The drawing under review shows one solid part. Ordinate dimensions are in mm from its lowest x, y, z. A direction names the side the tool comes from. Coordinates: 2 decimals unless noted, no trailing zeros. Order: outer loops, then holes, each group sorted by start corner. A loop starts at its lowest first (then second) coordinate and runs counter-clockwise, first axis right, second up. Notation, with made-up numbers: M 26.5,49.25 L 41.5,49.25 A26 ccw 41.5,70.25 Z; hole C 29.25,80.5 d2. An arc over 180 degrees is marked long. Answer as a JSON object with one key per item and string values.
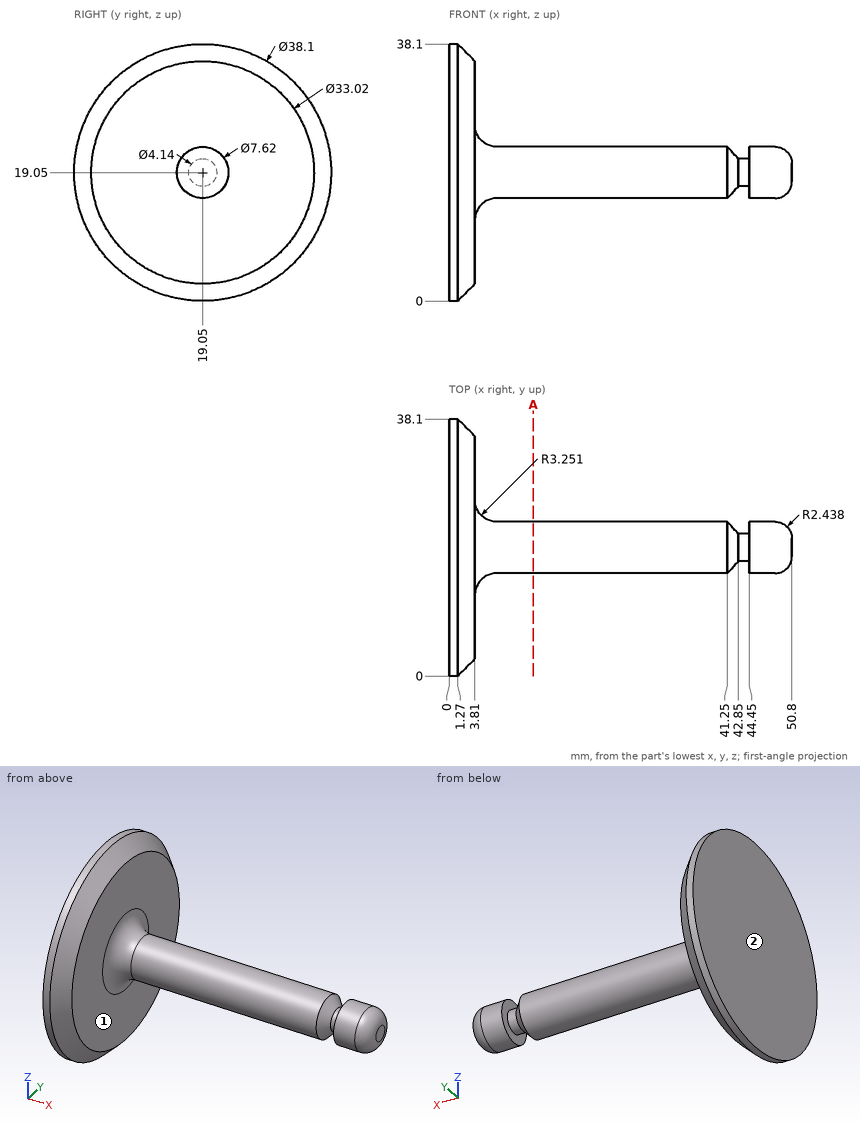
1) To check wall thickness, follow L1, parallel to X at y = 19.5, z = 34; L2, parallel to Z at x = 41, y = 19; L3, parallel to X at y = 24, z = 19. State the ranges of each line that lie inside material, in increasing order.
Taken from the geometry:
{"L1": "x = 0 to 3.81", "L2": "z = 15.24 to 22.86", "L3": "x = 0 to 4.59"}
2) Tool access review of the marked faces 1 and 2: name each direction out of +Z, -Z, +X, -X, +Y, -Y from which nothing blocks a thin tool from reaching the whole face with its end or side.
Taken from the geometry:
{"face 1": "+X", "face 2": "+Z, -Z, -X, +Y, -Y"}
3) Add section A-A (x = 12.5). State the section outline as (y, z) points.
Taken from the geometry:
{"outline": "C 19.05,19.05 d7.62"}
4) Insertion check: pin 1 Ø4 at (x, y) = (9.5, 15.5) entering from +Z; pin 2 Ø4 at (x, y) = (38.5, 14) entering from +Z (1 decimal); pin 3 Ø5 at (x, y) = (34.5, 19.5) entering from +Z. Each pin has a flat end and moves straight along its axis. Give the tip position at first contact, or say it passes through.
Taken from the geometry:
{"pin 1": "stops at z = 22.53", "pin 2": "stops at z = 21.3", "pin 3": "stops at z = 22.86"}
